Input: part model. Units: mm. Frame: model coordinates. A direction names the side the tool comes from. Round coordinates to 2 decimals unless told otherwise and drop trailing zeros. Write each loop counter-clockwise with the first axis right and the second up, starting at its lowest first coordinate (ties: lowest second). Pieces come first, ordered by that corner, then holes. Notation, with made-up numbers: (80, 3.5) - (121, 3.5) arc R30 ccw to (121, 31.5) - close; hole circle Ø8 at (77.25, 28). An arc over 180 degrees is marked (long way). Use one line per item in the form item = value.
```python
from build123d import *

# Parameters (mm, degrees)
SKETCH1_W           = 33
SKETCH1_H           = 20
BOSS_EXTRUDE1_DEPTH = 2
SKETCH2_R           = 2
CUT_EXTRUDE1_DEPTH  = 20.704060495
SKETCH3_R           = 2.5
BOSS_EXTRUDE2_DEPTH = 8
FILLET1_SIZE        = 2


with BuildPart() as part:
    # Sketch1 → Boss-Extrude1 (new, symmetric)
    with BuildSketch(Plane(origin=(0, 0, 0), x_dir=(1, 0, 0), z_dir=(0, 1, 0))):
        Rectangle(SKETCH1_W, SKETCH1_H)
    extrude(amount=BOSS_EXTRUDE1_DEPTH, both=True)

    # Sketch2 → Cut-Extrude1 (cut, through all)
    with BuildSketch(Plane(origin=(0, 2, 0), x_dir=(1, 0, 0), z_dir=(0, 1, 0))):
        with Locations(Location((-14, 4, 0), (0, 0, 270))):
            Circle(SKETCH2_R)
        with Locations(Location((-14, -4, 0), (0, 0, 270))):
            Circle(SKETCH2_R)
        with Locations(Location((14, -4, 0), (0, 0, 90))):
            Circle(SKETCH2_R)
        with Locations(Location((14, 4, 0), (0, 0, 90))):
            Circle(SKETCH2_R)
    extrude(amount=-CUT_EXTRUDE1_DEPTH, mode=Mode.SUBTRACT)

    # Sketch3 → Boss-Extrude2 (add)
    with BuildSketch(Plane(origin=(0, 2, 0), x_dir=(1, 0, 0), z_dir=(0, 1, 0))):
        with Locations(Location((0, 0, 0), (0, 0, 270))):
            Circle(SKETCH3_R)
    extrude(amount=BOSS_EXTRUDE2_DEPTH)

    # Fillet1
    # a fillet whose section is not a circle: 2 mm, written as the material it adds along each edge
    with BuildSketch(Plane(origin=(0, 2, 0), x_dir=(0, 0, 1), z_dir=(-1, 0, 0))) as fillet1_piece_1:
        with BuildLine():
            Bezier((2.5 + FILLET1_SIZE, 0), (2.5, 0), (2.5, FILLET1_SIZE), weights=[1, 0.141421356, 1])
            Line((2.5, FILLET1_SIZE), (2.5, 0))
            Line((2.5, 0), (2.5 + FILLET1_SIZE, 0))
        make_face()
    revolve(axis=Axis((0, 2, 0), (0, 1, 0)))


solid = part.part
```
(1) Cut plane D-D on y = 8. Output: boundary loops of the cut face in (x, z).
Derived:
outline = circle Ø5 at (0, 0)
(2) Draft query along X for faces 1 (the face through (-16.5, 0, 0)), 2 (the face through (0, 0, -10)), 3 (the face through (12.648, 0.028, -2.526)), 4 (the face through (-12.648, 0.028, 2.526)). Return one class per face: released by +X, released by -X, zero draft, split by the parting line, or undercut.
Derived:
face_1 = released by -X
face_2 = zero draft
face_3 = undercut
face_4 = undercut
(3) Material intervals for L1, parallel to X at y = -0.95, z = 4; L2, parallel to Z at x = 14, y = -0.1; L3, parallel to Z at x = 15, y = -1, sorted ascending.
Derived:
L1 = -16.5 to -16, -12 to 12, 16 to 16.5
L2 = -10 to -6, -2 to 2, 6 to 10
L3 = -10 to -5.73, -2.27 to 2.27, 5.73 to 10
(4) Access query for faces 5 (the face through (0, 2, -5)), 6 (the face through (0, 0, 10)). Directions: +Z, -Z, +X, -X, +Y, -Y. A direction counts if a zero-diameter tool reaches every point of the face in a straight line with its end or side. Return the directions, or none.
Derived:
face_5 = +Y
face_6 = +Z, +X, -X, +Y, -Y
(5) First-contact query: pin 1 Ø1 at (x, z) = (-7, 2.5) entering from +Y; pin 2 Ø1 at (x, y) = (-1.5, 7.5) entering from -Z; pin 3 Ø8 at (x, z) = (3, -7) entering from +Y. Flat tips, straight axial feed; report the tip coordinate or a pass-through.
Derived:
pin_1 = 2
pin_2 = -2.29
pin_3 = 2.64
(6) Cut plane C-C on z = -3. Count the separate pieces of the cut face and the enclosed holes in it, then the cut area to 3 significant figures.
Derived:
separate_pieces = 3
enclosed_holes = 0
area = 109 mm^2
(7) Cut plane B-B on y = 1. Output: boundary loops of the cut face in (x, z).
Derived:
outline = (-16.5, -10) - (16.5, -10) - (16.5, 10) - (-16.5, 10) - close; hole circle Ø4 at (-14, -4); hole circle Ø4 at (-14, 4); hole circle Ø4 at (14, -4); hole circle Ø4 at (14, 4)
(8) Cut plane A-A on x = -14. Output: boundary loops of the cut face in (y, z), then the cut area to 3 significant figures.
Derived:
outline = (-2, -10) - (2, -10) - (2, -6) - (-2, -6) - close; (-2, -2) - (2, -2) - (2, 2) - (-2, 2) - close; (-2, 6) - (2, 6) - (2, 10) - (-2, 10) - close
area = 48.0 mm^2
